Read the model definition and answer for the solid it produces. Units are mm, in the model's axes. Face numbers are marked on the shaded views. A direction names the side the tool comes from. Coordinates: 2 decimals unless noted, no trailing zeros. Write each loop counter-clockwise with the first axis right and the second up, starting at its lowest first coordinate (ties: lowest second). Pieces come first, ordered by that corner, then holes. Notation, with made-up numbers: M 58.25,82 L 88.25,82 A18 cw 88.25,111 Z; hole C 19.5,70 d3. An arc over 180 degrees is marked long. Use a Markdown table: item, result. Add a question column.
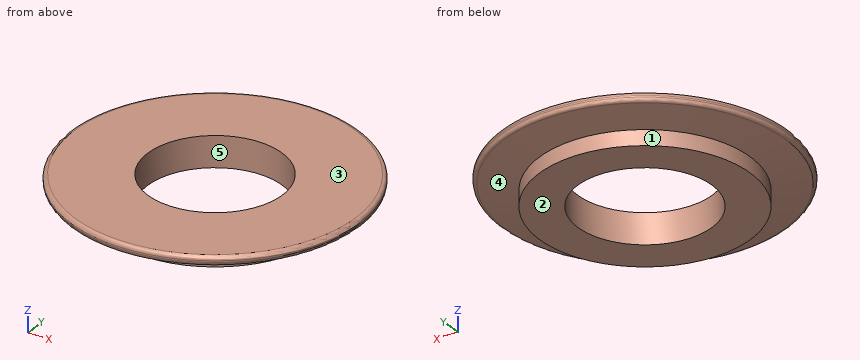
from build123d import *


with BuildPart() as f1:
    # F0 (on Right) → F1 (revolve)
    with BuildSketch(Plane.YZ):
        with BuildLine():
            Line((-27.5, 4), (-27.5, 0))
            Line((-27.5, 0), (-17.5, 0))
            Line((-17.5, 0), (-17.5, 8))
            Line((-17.5, 8), (-36.5, 8))
            ThreePointArc((-36.5, 8), (-37.207107, 7.707107), (-37.5, 7))
            Line((-37.5, 7), (-37.5, 6.590197))
            ThreePointArc((-37.5, 6.590197), (-37.265631, 5.946916), (-36.67238, 5.605167))
            Line((-36.67238, 5.605167), (-27.5, 4))
        make_face()
    revolve(axis=Axis((0, 0, 4), (0, 0, 1)))


solid = f1.part
Item 1: Consider probe 1 along X at (y, z) = (0, 6.5); probe 2 along X at (y, z) = (0, 1.75); probe 3 along Y at (x, z) = (1, 1.25). Determine where each line is inside the solid, lowest interval first.
Item 2: For the marked faces 1 and 2, determine the directions among +Z, -Z, +X, -X, +Y, -Y from which every point of the face is accessible in a straight line to the end or side of a thin tool.
Item 3: Determine the mould class of the marked faces 3, 4 and 5 for opening direction X: pulls with the +X half, pulls with the -X half, needs draft (parallel to the pull), parting line crosses it, or undercut.
Item 4: Find section C-C on z = 1. Give the vertices of the cut face in (x, y).
Item 5: Find section A-A on y = 0. Give the vertices of the cut face in (x, z).
Item 6: Each of these flat-tipped pins is pushed along its axis until it touches: pin 1 (2 mm diameter, centred on x = 17.5, z = 1.5, fed in from -Y); pin 2 (1 mm diameter, centred on x = 23, z = 6.5, fed in from -Y); pin 3 (2 mm diameter, centred on x = -27, z = 5.5, fed in from +Y). Where does it stop, or does it pass through?
Geometry says:
| question | item | result |
|---|---|---|
| 1 | probe 1 | x = -37.5 to -17.5, 17.5 to 37.5 |
| 1 | probe 2 | x = -27.5 to -17.5, 17.5 to 27.5 |
| 1 | probe 3 | y = -27.48 to -17.47, 17.47 to 27.48 |
| 2 | face 1 | -Z |
| 2 | face 2 | -Z, +X, -X, +Y, -Y |
| 3 | face 3 | needs draft |
| 3 | face 4 | parting line crosses it |
| 3 | face 5 | undercut |
| 4 | outline | C 0,0 d55; hole C 0,0 d35 |
| 5 | outline | M -37.5,6.59 A1 ccw -36.67,5.61 L -27.5,4 L -27.5,0 L -17.5,0 L -17.5,8 L -36.5,8 A1 ccw -37.5,7 Z; M 17.5,0 L 27.5,0 L 27.5,4 L 36.67,5.61 A1 ccw 37.5,6.59 L 37.5,7 A1 ccw 36.5,8 L 17.5,8 Z |
| 6 | pin 1 | stops at y = -22 |
| 6 | pin 2 | stops at y = -30 |
| 6 | pin 3 | stops at y = 26.65 |
